Geometry check sheet. Reference: the model listing, model coordinates, mm. Coordinates: 2 decimals unless noted, no trailing zeros. Answer as CSV lines item,"result". Start each with the question number.
from build123d import *

# Parameters (mm, degrees)
EXTRUDE_1_DEPTH     = 3
SKETCH_2_R          = 2.15
CUT_EXTRUDE_1_DEPTH = 3
SKETCH_3_R          = 1
CUT_EXTRUDE_2_DEPTH = 70


with BuildPart() as part:
    # 草图1 → 凸台-拉伸1 (new body)
    with BuildSketch(Plane.XY):
        Polygon((-51.0025, -60.127538713), (51.0025, -60.127538713), (51.0025, 19.872461287), (31.0025, 39.872461287), (-31.0025, 39.872461287), (-51.0025, 19.872461287), align=None)
    extrude(amount=-EXTRUDE_1_DEPTH)

    # 草图2 → 切除-拉伸1 (cut)
    with BuildSketch(Plane.XY):
        with Locations((-41.0025, 9.872461287)):
            Circle(SKETCH_2_R)
        with Locations((-41.0025, -50.127538713)):
            Circle(SKETCH_2_R)
        with Locations((41.0025, 9.872461287)):
            Circle(SKETCH_2_R)
        with Locations((41.0025, -50.127538713)):
            Circle(SKETCH_2_R)
    extrude(amount=-CUT_EXTRUDE_1_DEPTH, mode=Mode.SUBTRACT)

    # 草图3 → 切除-拉伸2 (cut)
    with BuildSketch(Plane(origin=(0, 0, -3), x_dir=(-1, 0, 0), z_dir=(0, 0, -1))):
        with Locations((-7.000166, 31.25)):
            Circle(SKETCH_3_R)
        with Locations((6.999834, 31.25)):
            Circle(SKETCH_3_R)
        with Locations((-7.000166, -48.75)):
            Circle(SKETCH_3_R)
        with Locations((6.999834, -48.75)):
            Circle(SKETCH_3_R)
    extrude(amount=-CUT_EXTRUDE_2_DEPTH, mode=Mode.SUBTRACT)


solid = part.part
Q1. Sectioned sample at A-A, the plane z = -0.45. Give the number of separate pieces and of enclosed holes in the cut face, then the cut area to 3 significant figures.
Q2. Release check for a two-part mould opening along Y. For faces 1 (the cylindrical face through (43.053, -49.482, -1.479)), 2 (the flat face through (41.142, 29.732, -1.479)), 3 (the cylindrical face through (43.053, 10.518, -1.479)), 4 (the flat face through (-51.002, -20, -1)) record: released by +Y, released by -Y, zero draft, split by the parting line, or undercut.
Q3. Thickness scan on L1, parallel to Y at x = 32, z = -1; L2, parallel to X at y = 31, z = -0.05; L3, parallel to Y at x = -46.5, z = -1.8. Record the ranges inside material, lowest first.
Geometry results:
1,separate pieces,"1"
1,enclosed holes,"8"
1,area,"9,730 mm^2"
2,face 1,"undercut"
2,face 2,"released by +Y"
2,face 3,"undercut"
2,face 4,"zero draft"
3,L1,"y = -60.13 to 38.87"
3,L2,"x = -39.87 to -7.97, -6.03 to 6.03, 7.97 to 39.87"
3,L3,"y = -60.13 to 24.37"
